Read the model definition and answer for the solid it produces. Units are mm, in the model's axes. A direction names the side the tool comes from. Give positions to 0.01 mm unless a question says otherwise; leave off trailing zeros. Loops run counter-clockwise (first coordinate to the right, second up) from the corner with the lowest first, then second, coordinate; pieces in that order, holes last.
(1) Which of the six approach directions +Z, -Z, +X, -X, +Y, -Y give full straight-line access (tool end or side, diameter ignored) to faces 5 (the face through (38.11, 0.165, -3.746)), 6 (the face through (2.4, 1.25, 4.2)), 7 (the face through (2.4, -1.25, 4.3)), 8 (the face through (0.99, -7.81, -1.73))?
(2) Find section A-A, the plane y = 0. Write down the section's boundary in (x, z), then the cut area to 3 significant figures.
(3) Straight lines are drawn through the part: probe 1 along X at (y, z) = (-1, 7); probe 2 along Y at (x, z) = (27, -0.25); probe 3 along Y at (x, z) = (36.5, -3). For each, find the intervals that lie inside material, in ascending order.
(4) Determine the mould class of faces 1 (the face through (0, 0, 0)), 2 (the face through (40, 0, 0)), 3 (the face through (37.36, -1.947, -2.539)), 4 (the face through (19.255, 1.126, 3.577)) for opening direction X: pulls with the +X half, pulls with the -X half, needs draft (parallel to the pull), parting line crosses it, or undercut.
(5) Find section D-D, the plane y = -6.25. Write down the section's boundary in (x, z).
(6) Find section C-C, the plane x = 12. Write down the section's boundary in (y, z).
(7) Find section B-B, the plane z = 0. Write down the section's boundary in (x, y).
(8) Each of these flat-tipped pins is pushed along its axis until it touches: P1, Ø3, axis at x = 23.5, z = 0, coming from the +Y side; P2, Ø2, axis at x = 21, y = -3, coming from the -Z side; P3, Ø1.5, axis at x = 10.5, z = -3.5, coming from the -Y side. Where does it stop, or does it pass through?
```python
from build123d import *

# Parameters (mm, degrees)
F3_DEPTH = 1.5
F5_DEPTH = 25
F6_R     = 1.5


with BuildPart() as f1:
    # F0 (on Front) → F1 (revolve)
    with BuildSketch(Plane.XZ):
        Polygon((0, 8), (0, 0), (40, 0), (40, 3.75), (37.73, 3.75), (37.73, 3.2), (37, 3.2), (37, 3.75), (2, 3.75), (2, 8), align=None)
    revolve(axis=Axis((20, 0, 0), (-1, 0, 0)))

    # F2 (on face) → F3 (join, symmetric)
    with BuildSketch(Plane.YZ.offset(2)):
        with BuildLine():
            Line((-1.25, 6.076651), (-1.25, 3.535534))
            ThreePointArc((-1.25, 3.535534), (0, 3.75), (1.25, 3.535534))
            Line((1.25, 3.535534), (1.25, 6.076651))
            Line((1.25, 6.076651), (-1.25, 6.076651))
        make_face()
    extrude(amount=F3_DEPTH, both=True)

    # F4 (on face) → F5 (cut)
    with BuildSketch(Plane(origin=(0, 1.25, 0), x_dir=(-1, 0, 0), z_dir=(0, 1, 0))):
        Polygon((-3.5, 3.535534), (-2, 6.076651), (-3.5, 6.076651), align=None)
    extrude(amount=-F5_DEPTH, mode=Mode.SUBTRACT)

    # F6
    f6_edges = [f1.edges().sort_by_distance(p)[0] for p in [
        (40, 0, -3.75),
    ]]
    fillet(f6_edges, radius=F6_R)


solid = f1.part
```
Entries:
1. face 5: +X
1. face 6: +Z, +X, +Y
1. face 7: +Z, +X, -Y
1. face 8: +X, -X
2. outline: (0, -8) - (2, -8) - (2, -3.75) - (37, -3.75) - (37, -3.2) - (37.73, -3.2) - (37.73, -3.75) - (38.5, -3.75) arc R1.5 ccw to (40, -2.25) - (40, 2.25) arc R1.5 ccw to (38.5, 3.75) - (37.73, 3.75) - (37.73, 3.2) - (37, 3.2) - (37, 3.75) - (3.5, 3.75) - (3.5, 3.54) - (2, 6.08) - (2, 8) - (0, 8) - close
2. area: 317 mm2
3. probe 1: x = 0 to 2
3. probe 2: y = -3.74 to 3.74
3. probe 3: y = -2.25 to 2.25
4. face 1: pulls with the -X half
4. face 2: pulls with the +X half
4. face 3: undercut
4. face 4: needs draft
5. outline: (0, -4.99) - (2, -4.99) - (2, 4.99) - (0, 4.99) - close
6. outline: circle Ø7.5 at (0, 0)
7. outline: (0, -8) - (2, -8) - (2, -3.75) - (37, -3.75) - (37, -3.2) - (37.73, -3.2) - (37.73, -3.75) - (38.5, -3.75) arc R1.5 ccw to (40, -2.25) - (40, 2.25) arc R1.5 ccw to (38.5, 3.75) - (37.73, 3.75) - (37.73, 3.2) - (37, 3.2) - (37, 3.75) - (2, 3.75) - (2, 8) - (0, 8) - close
8. P1: stops at y = 3.75
8. P2: stops at z = -3.17
8. P3: stops at y = -2.55
